Verification items for this drawing (mm, ordinates from the low corner). Coordinates: 2 decimals unless noted, no trailing zeros. Order: outer loops, then holes, each group sorted by start corner. A loop starts at its lowest first (then second) coordinate and runs counter-clockwise, first axis right, second up. Notation, with made-up numbers: (66.25, -26) -> (87.25, -26) arc R16 ccw to (87.25, -9) -> close; hole circle Ø11 at (-19.5, 23.5). An arc over 180 degrees is marked (long way). Write item = value, one per line. Start each with the question number.
1. Thickness scan on line 1 along Z through (x, y) = (56, 0.45); line 2 along X through (y, z) = (1.4, 3.25); line 3 along X through (y, z) = (1.3, 3.75). Record the ranges inside material, lowest first. Write a range as from..to.
2. Cross-section at A-A on x = 7. Record the cut outline in (y, z), plus the area to 3 significant figures.
3. Cross-section at B-B on y = 0.9. Record the cut outline in (x, z).
4. Cross-section at C-C on z = 4. Record the cut outline in (x, y), plus the area to 3 significant figures.
5. Go/stop test with a flat-tipped pin: P1, Ø1.6, axis at x = 31.5, z = 4, coming from the +Y side. Record where the tip stops, or that it passes through.
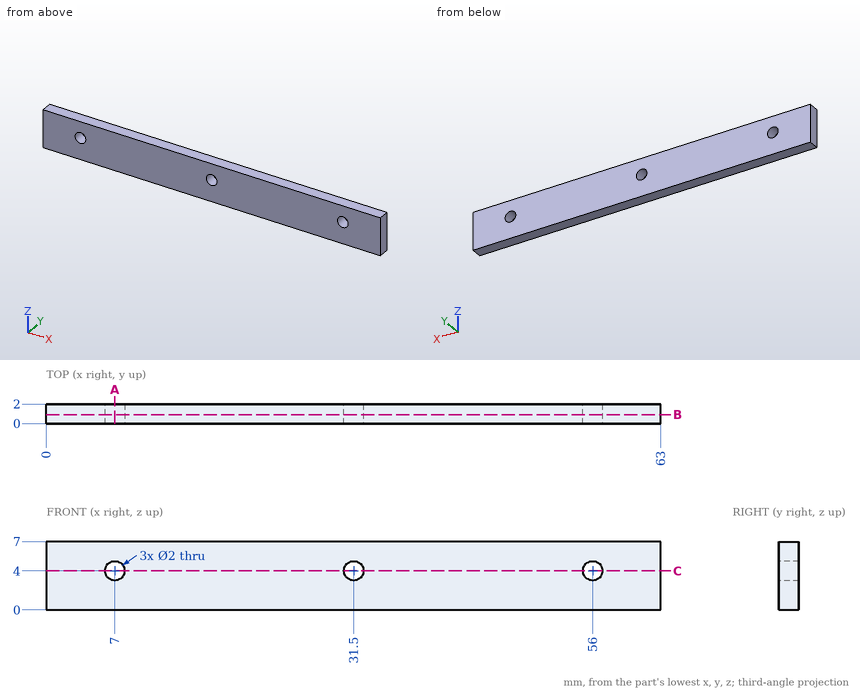
Worked out:
q1.line_1 = 0..3, 5..7
q1.line_2 = 0..6.34, 7.66..30.84, 32.16..55.34, 56.66..63
q1.line_3 = 0..6.03, 7.97..30.53, 32.47..55.03, 56.97..63
q2.outline = (0, 0) -> (2, 0) -> (2, 3) -> (0, 3) -> close; (0, 5) -> (2, 5) -> (2, 7) -> (0, 7) -> close
q2.area = 10.0 mm²
q3.outline = (0, 0) -> (63, 0) -> (63, 7) -> (0, 7) -> close; hole circle Ø2 at (7, 4); hole circle Ø2 at (31.5, 4); hole circle Ø2 at (56, 4)
q4.outline = (0, 0) -> (6, 0) -> (6, 2) -> (0, 2) -> close; (8, 0) -> (30.5, 0) -> (30.5, 2) -> (8, 2) -> close; (32.5, 0) -> (55, 0) -> (55, 2) -> (32.5, 2) -> close; (57, 0) -> (63, 0) -> (63, 2) -> (57, 2) -> close
q4.area = 114 mm²
q5.P1 = through
